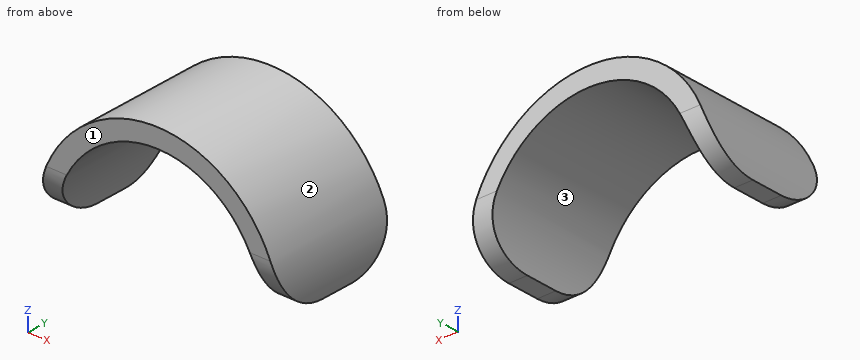
Autodesk Inventor part; units mm, degrees
ref_plane "YZ Plane" through (0, 0, 0) normal (1, 0, 0) x (0, 1, 0)
ref_plane "XZ Plane" through (0, 0, 0) normal (0, 1, 0) x (-1, 0, 0)
ref_plane "XY Plane" through (0, 0, 0) normal (0, 0, 1) x (1, 0, 0)
sketch "Sketch1" plane through (0, 0, 0) normal (0, 1, 0) x (-1, 0, 0)
  arc A0 (24.13, 0) -> (-24.13, 0) centre (0, 0) ccw
  arc A1 (20.447, 0) -> (-20.447, 0) centre (0, 0) ccw
  line L0 (24.13, 0) -> (-24.13, 0)
  dimension "d0" = 48.26
  dimension "d1" = 40.894
extrude "Extrusion1" add sketch "Sketch1" along normal mid plane 25.4 contours L0 A1 A0
fillet "Fillet1" radius 9.525 4 edges at (-22.2885, 12.7, 0) (-22.2885, -12.7, 0) (22.2885, -12.7, 0) (22.2885, 12.7, 0)
properties part number "FE-120-004 Pivot Hardstop" material "PVC-Piping"
Read the model definition and answer for the solid it produces. Units are mm, in the model's axes. Face numbers are marked on the shaded views. Coordinates: 2 decimals unless noted, no trailing zeros. Write each loop counter-clockwise with the first axis right and the second up, starting at its lowest first coordinate (ties: lowest second). Pieces come first, ordered by that corner, then holes. Notation, with made-up numbers: (42, -35) -> (67, -35) arc R25 ccw to (67, -10) -> close; hole circle Ø9 at (23.5, 31). An arc over 180 degrees is marked (long way). Write item = value, one per line.
(1) Given pin 1 Ø10 at (x, y) = (-10, 5) entering from +Z; pin 2 Ø2 at (y, z) = (-6.5, 21.5) entering from -X; pin 3 Ø6 at (y, z) = (8.5, 14.5) entering from -X, each flat-ended and moving along its own axis, determine where each tip first touches the part or whether it passes through.
From the geometry:
pin_1 = 23.61
pin_2 = -12.73
pin_3 = -21.21
(2) Section C-C on z = 16.5 is taken. Write down the section's boundary in (x, y).
From the geometry:
outline = (-17.61, -12.7) -> (-12.08, -12.7) -> (-12.08, 12.7) -> (-17.61, 12.7) -> close; (12.08, -12.7) -> (17.61, -12.7) -> (17.61, 12.7) -> (12.08, 12.7) -> close
(3) Section A-A on z = 5 is taken. Write down the section's boundary in (x, y), plus the area to 3 significant figures.
From the geometry:
outline = (-23.61, -11.56) -> (-19.83, -11.56) -> (-19.83, 11.56) -> (-23.61, 11.56) -> close; (19.83, -11.56) -> (23.61, -11.56) -> (23.61, 11.56) -> (19.83, 11.56) -> close
area = 175 mm2
(4) Section B-B on x = 0 is taken. Write down the section's boundary in (y, z), plus the area to 3 significant figures.
From the geometry:
outline = (-12.7, 20.45) -> (12.7, 20.45) -> (12.7, 24.13) -> (-12.7, 24.13) -> close
area = 93.5 mm2
(5) Section D-D on y = -10.75 is taken. Write down the section's boundary in (x, z).
From the geometry:
outline = (-23.84, 3.75) -> (-20.1, 3.75) arc R20.45 cw to (20.1, 3.75) -> (23.84, 3.75) arc R24.13 ccw to start
(6) For a pull along X with two mould halves and no side action, classify the marked faces 1, 2 and 3 as +X half, -X half, draft (parallel to the pull), parting line (faces both ways), or undercut.
From the geometry:
face_1 = draft
face_2 = parting line
face_3 = undercut
(7) Straight lines are drawn through the part: L1, parallel to X at y = 1.5, z = 11.5; L2, parallel to X at y = 3.75, z = 14; L3, parallel to X at y = -3, z = 21. For each, find the intervals that lie inside material, in ascending order. Write a range as from..to.
From the geometry:
L1 = -21.21..-16.91, 16.91..21.21
L2 = -19.65..-14.9, 14.9..19.65
L3 = -11.89..11.89
